Verification items for the finished model (mm, model axes). Give positions to 0.01 mm unless a question says otherwise; leave off trailing zeros. Order: outer loops, then holes, each group sorted by start corner. A loop starts at its lowest first (then second) coordinate and runs counter-clockwise, first axis right, second up. Notation, with made-up numbers: (-31, -37) - (11, -37) arc R19 cw to (11, -20) - close; hole circle Ø1 at (53.25, 32). An arc over 180 degrees is marked (long way). Answer as a JSON object with one key per item and string values.
Autodesk Inventor part; units mm, degrees
ref_plane "YZ Plane" through (0, 0, 0) normal (1, 0, 0) x (0, 1, 0)
ref_plane "XZ Plane" through (0, 0, 0) normal (0, 1, 0) x (-1, 0, 0)
ref_plane "XY Plane" through (0, 0, 0) normal (0, 0, 1) x (1, 0, 0)
sketch "Sketch1" plane through (0, 0, 0) normal (0, 1, 0) x (-1, 0, 0)
  line L0 (65, 90) -> (35, 90)
  line L1 (35, 90) -> (35, -310)
  line L2 (35, -310) -> (65, -310)
  line L3 (65, -310) -> (65, 90)
  line L4 (50, 90) -> (50, -310) construction
  circle A0 centre (50, 70) radius 6
  circle A1 centre (50, -290) radius 6
  point P0 (0, 0)
  dimension "d0" = 30
  dimension "d1" = 400
  dimension "d2" = 35
  dimension "d3" = 90
  dimension "d6" = 12
  dimension "d7" = 12
  dimension "d8" = 20
  dimension "d9" = 20
extrude "Extrusion1" add sketch "Sketch1" along normal blind 3
properties part number "rig_connector_long"
(1) Section check A-A (z = -290). Record the cut outline in (x, y), then the cut area to 3 significant figures.
Computed values:
{"outline": "(-65, 0) - (-56, 0) - (-56, 3) - (-65, 3) - close; (-44, 0) - (-35, 0) - (-35, 3) - (-44, 3) - close", "area": "54.0 mm²"}
(2) Release check for a two-part mould opening along X. For faces 1 (the cylindrical face through (-49.22, 1.48, 64.05)), 2 (the cylindrical face through (-53.226, 1.479, -295.059)), 3 (the flat face through (-50, 0, -107)) record: pulls with the +X half, pulls with the -X half, needs draft (parallel to the pull), parting line crosses it, or undercut.
Computed values:
{"face 1": "undercut", "face 2": "undercut", "face 3": "needs draft"}
(3) Section check B-B (y = 1.95). Record the cut outline in (x, z).
Computed values:
{"outline": "(-65, -310) - (-35, -310) - (-35, 90) - (-65, 90) - close; hole circle Ø12 at (-50, -290); hole circle Ø12 at (-50, 70)"}
(4) Material ranges on line 1 along Z through (x, y) = (-50, 0.7); line 2 along Z through (x, y) = (-52.25, 0.95); line 3 along X through (y, z) = (2, -290), recorded low to high. Write a range as [from, to].
Computed values:
{"line 1": "z = [-310, -296], [-284, 64], [76, 90]", "line 2": "z = [-310, -295.56], [-284.44, 64.44], [75.56, 90]", "line 3": "x = [-65, -56], [-44, -35]"}
(5) Section check C-C (x = -50). Record the cut outline in (y, z), then the cut area to 3 significant figures.
Computed values:
{"outline": "(0, -310) - (3, -310) - (3, -296) - (0, -296) - close; (0, -284) - (3, -284) - (3, 64) - (0, 64) - close; (0, 76) - (3, 76) - (3, 90) - (0, 90) - close", "area": "1,130 mm²"}
